```python
from build123d import *

# Parameters (mm, degrees)
SKETCH1_R     = 2
LENGTH_DEPTH  = 43.18
SKETCH2_R     = 4.5
CAP_DEPTH     = 2
HEX_CUT_DEPTH = 1.238
CHAMFER1_SIZE = 1.905


with BuildPart() as part:
    # Sketch1 → Length (new body)
    with BuildSketch(Plane(origin=(0, 0, 0), x_dir=(1, 0, 0), z_dir=(0, 1, 0))):
        with Locations(Location((0, 0, 0), (0, 0, 270))):
            Circle(SKETCH1_R)
    extrude(amount=LENGTH_DEPTH)

    # Sketch2 → Cap (add)
    with BuildSketch(Plane(origin=(0, 43.18, 0), x_dir=(1, 0, 0), z_dir=(0, 1, 0))):
        with Locations(Location((0, 0, 0), (0, 0, 270))):
            Circle(SKETCH2_R)
    extrude(amount=CAP_DEPTH)

    # Sketch3 → Hex cut (cut)
    with BuildSketch(Plane(origin=(0, 45.18, 0), x_dir=(1, 0, 0), z_dir=(0, 1, 0))):
        Polygon((0, 3), (-2.598076211, 1.5), (-2.598076211, -1.5), (0, -3), (2.598076211, -1.5), (2.598076211, 1.5), align=None)
    extrude(amount=-HEX_CUT_DEPTH, mode=Mode.SUBTRACT)

    # Chamfer1
    chamfer1_edges = [part.edges().sort_by_distance(p)[0] for p in [
        (0, 43.18, -4.5),
    ]]
    chamfer(chamfer1_edges, length=CHAMFER1_SIZE)


solid = part.part
```
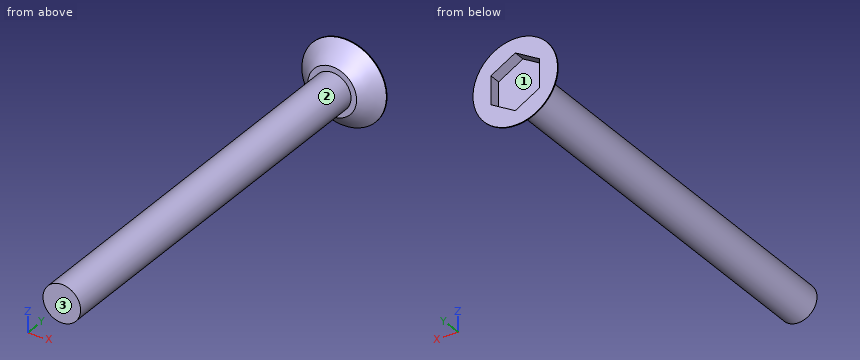
CAD build for the part. Positions are in the model's coordinates, mm. Face numbers are marked on the shaded views. Round coordinates to 2 decimals unless told otherwise and drop trailing zeros. Order: outer loops, then holes, each group sorted by start corner. A loop starts at its lowest first (then second) coordinate and runs counter-clockwise, first axis right, second up. Notation, with made-up numbers: (-37, -4) - (-27, -4) arc R21 ccw to (-27, 30) - close; hole circle Ø4 at (58, 2). An arc over 180 degrees is marked (long way). Answer in a Markdown table with one row per item. Add a question column.
(1) Drop flat-ended pins along their axis: pin 1 Ø5 at (y, z) = (28.5, -1.5) entering from +X; pin 2 Ø3 at (y, z) = (20, -3) entering from +X; pin 3 Ø1 at (x, y) = (3.5, 5) entering from +Z; pin 4 Ø0.6 at (y, z) = (44.5, -0.5) entering from +X. Give the stop position or say it passes through.
(2) Band-saw the part on A-A on z = 0. List the corners of the cut face in (x, y) (3 decimals).
(3) Mould opens along X. For the marked faces 1, 2 and 3 say: +X half, -X half, draft (parallel to the pull), parting line (faces both ways), or undercut.
(4) Band-saw the part on B-B on y = 39. List the corners of the cut face in (x, z).
(5) Probe L1, parallel to Y at x = -1.5, z = 1.75; L2, parallel to Y at x = 0.5, z = 0.5; L3, parallel to Z at x = 1.5, y = 7.5. List the from-to ranges inside material, lowest first. Write a range as [from, to].
Data:
| question | item | result |
|---|---|---|
| 1 | pin 1 | stops at x = 2 |
| 1 | pin 2 | stops at x = 1.32 |
| 1 | pin 3 | passes through |
| 1 | pin 4 | stops at x = 4.19 |
| 2 | outline | (-4.5, 45.085) - (-2.595, 43.18) - (-2, 43.18) - (-2, 0) - (2, 0) - (2, 43.18) - (2.595, 43.18) - (4.5, 45.085) - (4.5, 45.18) - (2.598, 45.18) - (2.598, 43.942) - (-2.598, 43.942) - (-2.598, 45.18) - (-4.5, 45.18) - close |
| 3 | face 1 | undercut |
| 3 | face 2 | parting line |
| 3 | face 3 | draft |
| 4 | outline | circle Ø4 at (0, 0) |
| 5 | L1 | y = [43.18, 43.94] |
| 5 | L2 | y = [0, 43.94] |
| 5 | L3 | z = [-1.32, 1.32] |
